Input: part model. Units: mm. Frame: model coordinates. A direction names the side the tool comes from. Round coordinates to 2 decimals unless told otherwise and drop trailing zeros. Loops run counter-clockwise (first coordinate to the right, second up) from the corner with the lowest first, then second, coordinate; pieces in that order, holes last.
(1) Cut plane C-C, the plane y = 48. Output: boundary loops of the cut face in (x, z).
(2) Cut plane D-D, the plane x = 36. Output: boundary loops of the cut face in (y, z).
(3) First-contact query: pin 1 Ø9 at (x, y) = (12.5, 56) entering from +Z; pin 2 Ø4.5 at (x, z) = (47.5, 25) entering from -Y; pin 3 Ø20 at (y, z) = (58.5, 25) entering from +X. Flat tips, straight axial feed; report the tip coordinate or a pass-through.
(4) Access query for faces 4 (the face through (46, 64.5, 3)), 5 (the face through (-4, -62, 1.8)), 6 (the face through (40.4, 62, 3)), 7 (the face through (0, 46.5, 23)). Directions: +Z, -Z, +X, -X, +Y, -Y. A direction counts if a zero-diameter tool reaches every point of the face in a straight line with its end or side. Return the directions, or none.
(5) Cut plane A-A, the plane x = -43.35. Output: boundary loops of the cut face in (y, z).
(6) Cut plane B-B, the plane z = 10.5. Output: boundary loops of the cut face in (x, y).
(7) Draft query along X for faces 1 (the face through (-44.16, 58.45, 3.45)), 2 (the face through (49.15, -1, 19)), 3 (the face through (-24, -64.5, 1)). Return one class per face: released by +X, released by -X, zero draft, split by the parting line, or undercut.
(8) Line query: line 1 (Y direction, x = -43.35, z = 2.25); line 2 (Y direction, x = 33, z = 22); line 3 (X direction, y = 58, z = 30.5). Output: solid intervals per line, ascending.
from build123d import *

# Parameters (mm, degrees)
SKETCH_1_W          = 98.3
SKETCH_1_H          = 129
EXTRUDE_1_DEPTH     = 38
SKETCH_2_W          = 96.5
SKETCH_2_H          = 18
CUT_EXTRUDE_1_DEPTH = 31
SKETCH_3_W          = 96.5
SKETCH_3_H          = 5
CUT_EXTRUDE_2_DEPTH = 36.2
SKETCH_4_R          = 1.75
CUT_EXTRUDE_3_DEPTH = 90.554299171


with BuildPart() as part:
    # 草图1 → 凸台-拉伸1 (new body)
    with BuildSketch(Plane.XY):
        Rectangle(SKETCH_1_W, SKETCH_1_H)
    extrude(amount=EXTRUDE_1_DEPTH)

    # 草图2 → 切除-拉伸1 (cut)
    with BuildSketch(Plane.XY.offset(38)):
        with Locations((0.9, 55.5)):
            Rectangle(SKETCH_2_W, SKETCH_2_H)
    extrude(amount=-CUT_EXTRUDE_1_DEPTH, mode=Mode.SUBTRACT)

    # 草图3 → 切除-拉伸2 (cut)
    with BuildSketch(Plane.XY.offset(38)):
        with Locations((0.9, -62)):
            Rectangle(SKETCH_3_W, SKETCH_3_H)
    extrude(amount=-CUT_EXTRUDE_2_DEPTH, mode=Mode.SUBTRACT)

    # 草图4 → 切除-拉伸3 (cut, through all)
    with BuildSketch(Plane(origin=(0, 0, 0), x_dir=(-1, 0, 0), z_dir=(0, 0, -1))):
        with Locations((43.35, 60)):
            Circle(SKETCH_4_R)
        with BuildLine():
            Line((-40.4, 60), (-40.4, 64.5))
            Line((-40.4, 64.5), (-43.9, 64.5))
            Line((-43.9, 64.5), (-43.9, 60))
            ThreePointArc((-43.9, 60), (-42.15, 58.25), (-40.4, 60))
        make_face()
        with BuildLine():
            Line((-40.4, -60.25), (-40.4, -64.5))
            Line((-40.4, -64.5), (-43.9, -64.5))
            Line((-43.9, -64.5), (-43.9, -60.25))
            ThreePointArc((-43.9, -60.25), (-42.15, -58.5), (-40.4, -60.25))
        make_face()
        with BuildLine():
            Line((41.6, -61.5), (41.6, -60.25))
            ThreePointArc((41.6, -60.25), (43.35, -58.5), (45.1, -60.25))
            Line((45.1, -60.25), (45.1, -61.5))
            ThreePointArc((45.1, -61.5), (43.35, -63.25), (41.6, -61.5))
        make_face()
    extrude(amount=-CUT_EXTRUDE_3_DEPTH, mode=Mode.SUBTRACT)


solid = part.part
Reported:
1. outline: (-49.15, 0) - (49.15, 0) - (49.15, 7) - (-47.35, 7) - (-47.35, 38) - (-49.15, 38) - close
2. outline: (-64.5, 0) - (64.5, 0) - (64.5, 7) - (46.5, 7) - (46.5, 38) - (-59.5, 38) - (-59.5, 1.8) - (-64.5, 1.8) - close
3. pin 1: stops at z = 7
3. pin 2: stops at y = -59.5
3. pin 3: stops at x = -47.35
4. face 4: +Z, -Z, +X, -X, +Y
4. face 5: +Z, +X, -Y
4. face 6: +Z, -Z, +Y
4. face 7: +Z, +X, +Y
5. outline: (-64.5, 0) - (-63.25, 0) - (-63.25, 1.8) - (-64.5, 1.8) - close; (-58.5, 0) - (58.25, 0) - (58.25, 7) - (46.5, 7) - (46.5, 38) - (-58.5, 38) - close; (61.75, 0) - (64.5, 0) - (64.5, 7) - (61.75, 7) - close
6. outline: (-49.15, -64.5) - (-47.35, -64.5) - (-47.35, -59.5) - (-44.93, -59.5) arc R1.75 cw to (-41.77, -59.5) - (40.57, -59.5) arc R1.75 cw to (43.73, -59.5) - (49.15, -59.5) - (49.15, 46.5) - (-47.35, 46.5) - (-47.35, 64.5) - (-49.15, 64.5) - close
7. face 1: undercut
7. face 2: released by +X
7. face 3: zero draft
8. line 1: y = -58.5 to 58.25, 61.75 to 64.5
8. line 2: y = -59.5 to 46.5
8. line 3: x = -49.15 to -47.35
